from build123d import *

# Parameters (mm, degrees)
F0_W     = 60
F0_H     = 10
F1_DEPTH = 10
F2_W     = 52.573141
F2_H     = 1.6
F3_DEPTH = 5
F4_W     = 11
F4_H     = 4.2
F5_DEPTH = 10.001


with BuildPart() as f1:
    # F0 (on Front) → F1 (new body)
    with BuildSketch(Plane.XZ):
        with Locations((5.357166, -16.956311)):
            Rectangle(F0_W, F0_H)
    extrude(amount=F1_DEPTH)

    # F2 (on face) → F3 (cut)
    with BuildSketch(Plane.XY.offset(-11.956311)):
        with Locations((5.024185, -5)):
            Rectangle(F2_W, F2_H)
    extrude(amount=-F3_DEPTH, mode=Mode.SUBTRACT)

    # F4 (on face) → F5 (cut, through all)
    with BuildSketch(Plane.XY.offset(-11.956311)):
        with Locations((5.357166, -7.9)):
            Rectangle(F4_W, F4_H)
    extrude(amount=-F5_DEPTH, mode=Mode.SUBTRACT)


solid = f1.part
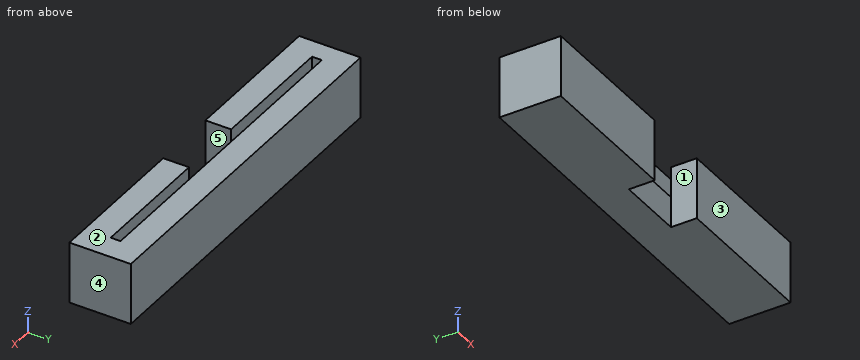
Input: part model. Units: mm. Frame: model coordinates. Face numbers are marked on the shaded views. A direction names the side the tool comes from. Round coordinates to 2 decimals unless told otherwise and drop trailing zeros. Loops run counter-clockwise (first coordinate to the right, second up) from the corner with the lowest first, then second, coordinate; pieces in that order, holes last. Notation, with made-up numbers: M -11.75,62 L 40.25,62 A26 ccw 40.25,85 Z; hole C 86.5,-14 d4. An arc over 180 degrees is marked long. Answer as CSV lines item,"result". Start each with the question number.
(1) Section C-C, the plane y = -5.25. Output: boundary loops of the cut face in (x, z).
(2) Section A-A, the plane y = -8.5. Output: boundary loops of the cut face in (x, z), plus the area to 3 significant figures.
(3) First-contact query: pin 1 (1.5 mm diameter, centred on x = 2.5, z = -18.5, fed in from -Y). Flat tip, straight axial feed; report the tip coordinate or a pass-through.
(4) Reachability of the marked faces 1 and 2 from +Z, -Z, +X, -X, +Y, -Y: full face, straight path, thin tool, end or side. Return the list, or none.
(5) Line query: line 1 (X direction, y = -7.75, z = -15.5); line 2 (X direction, y = -4.5, z = -16); line 3 (Y direction, x = -21, z = -16.75). Output: solid intervals per line, ascending. Write a range as [from, to].
(6) Section B-B, the plane z = -19.5. Output: boundary loops of the cut face in (x, y).
(7) Draft query along X for the marked faces 3, 4 and 5. Return one class per face: released by +X, released by -X, zero draft, split by the parting line, or undercut.
(8) Section D-D, the plane z = -15.5. Output: boundary loops of the cut face in (x, y), plus the area to 3 significant figures.
Values found:
1,outline,"M -24.64,-21.96 L 35.36,-21.96 L 35.36,-11.96 L 31.31,-11.96 L 31.31,-16.96 L -21.26,-16.96 L -21.26,-11.96 L -24.64,-11.96 Z"
2,outline,"M -24.64,-21.96 L -0.14,-21.96 L -0.14,-11.96 L -24.64,-11.96 Z; M 10.86,-21.96 L 35.36,-21.96 L 35.36,-11.96 L 10.86,-11.96 Z"
2,area,"490 mm²"
3,pin 1,"stops at y = -5.8"
4,face 1,"+Z, -Z, -Y"
4,face 2,"+Z, +X, -X, +Y, -Y"
5,line 1,"x = [-24.64, -0.14], [10.86, 35.36]"
5,line 2,"x = [-24.64, -21.26], [31.31, 35.36]"
5,line 3,"y = [-10, -5.8], [-4.2, 0]"
6,outline,"M -24.64,-10 L -0.14,-10 L -0.14,-5.8 L 10.86,-5.8 L 10.86,-10 L 35.36,-10 L 35.36,0 L -24.64,0 Z"
7,face 3,"zero draft"
7,face 4,"released by +X"
7,face 5,"undercut"
8,outline,"M -24.64,-10 L -0.14,-10 L -0.14,-5.8 L -21.26,-5.8 L -21.26,-4.2 L 31.31,-4.2 L 31.31,-5.8 L 10.86,-5.8 L 10.86,-10 L 35.36,-10 L 35.36,0 L -24.64,0 Z"
8,area,"470 mm²"
